Part print with two shaded views. Sizes in mm from the minimum x, y, z corner. Coordinates: 2 decimals unless noted, no trailing zeros. Loops run counter-clockwise (first coordinate to the right, second up) from the corner with the lowest first, then second, coordinate; pieces in that order, holes last. Notation, with made-up numbers: (41, 22.25) - (75, 22.25) arc R30 cw to (75, 61.25) - close; hole circle Ø10 at (9, 6.5). An arc over 180 degrees is marked (long way). Write each question's results on one line, items separated by ' | '. Start each with the question number.
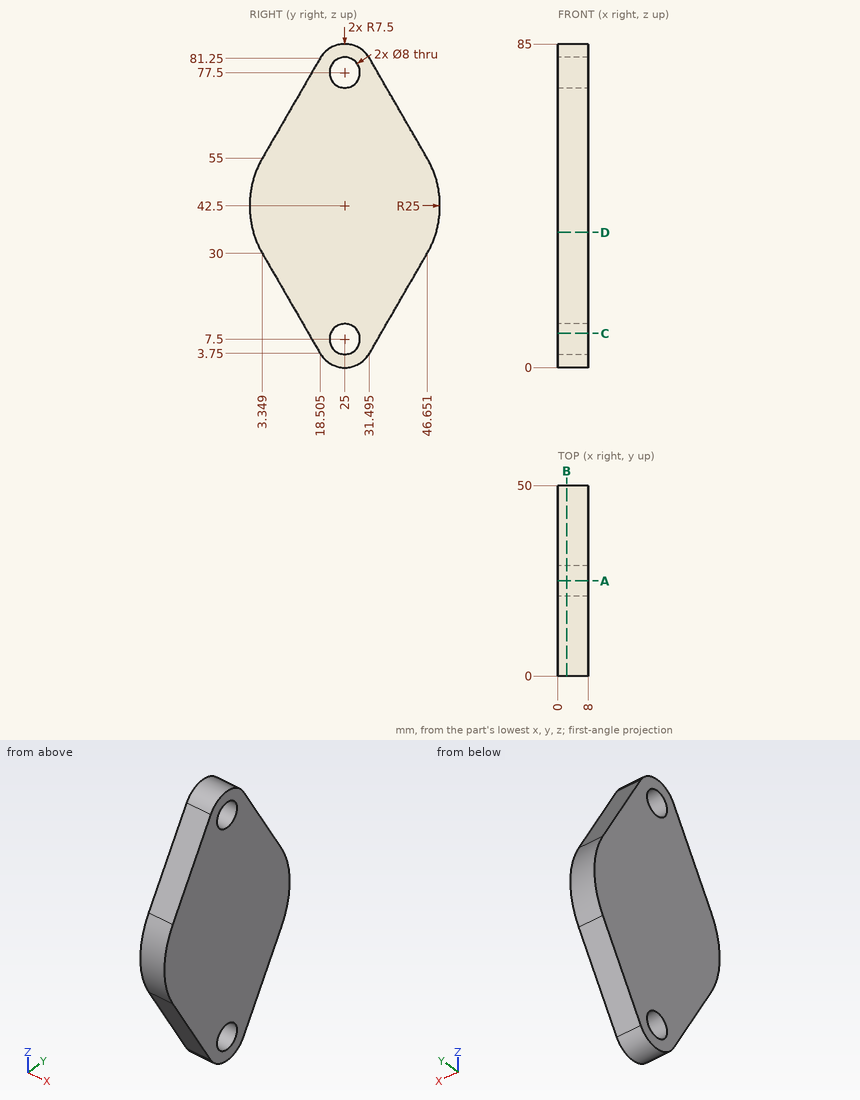
Q1. Cut at C-C (z = 9). List the corners of the cut face in (x, y), and give its area (3 significant figures).
Q2. Cut at B-B (x = 2.25). State how many separate pieces and enclosed holes the cut face has, and give its area (3 significant figures).
Q3. Cut at A-A (y = 25). List the corners of the cut face in (x, z).
Q4. Pin check, flat tips, straight feed: pin 1 (2 mm diameter, centred on x = 3, y = 43.5, fed in from +Z); pin 2 (2 mm diameter, centred on x = 1, z = 23, fed in from -Y); pin 3 (2 mm diameter, centred on x = 3.5, y = 13, fed in from +Z); pin 4 (10.5 mm diameter, centred on y = 25, z = 7.5, fed in from -X). Stop position of each tip, or through.
Q5. Drill centre lines: L1, parallel to Y at x = 5.75, z = 7.5; L2, parallel to Z at x = 2.5, y = 26.5; L3, parallel to Y at x = 4, z = 4.5 (1 decimal). Where is each one in solid material? Low to high. Write a range as from..to.
Q6. Cut at D-D (z = 35.5). List the corners of the cut face in (x, y).
Check result:
1) outline: (0, 15.47) - (8, 15.47) - (8, 21.29) - (0, 21.29) - close; (0, 28.71) - (8, 28.71) - (8, 34.53) - (0, 34.53) - close | area: 93.1 mm²
2) separate pieces: 1 | enclosed holes: 2 | area: 2,640 mm²
3) outline: (0, 0) - (8, 0) - (8, 3.5) - (0, 3.5) - close; (0, 11.5) - (8, 11.5) - (8, 73.5) - (0, 73.5) - close; (0, 81.5) - (8, 81.5) - (8, 85) - (0, 85) - close
4) pin 1: z = 62.19 | pin 2: y = 6.81 | pin 3: z = 73.45 | pin 4: x = 0
5) L1: 16.34..21, 29..33.66 | L2: 0.15..3.79, 11.21..73.79, 81.21..84.85 | L3: 18.1..22.4, 27.6..31.9
6) outline: (0, 1) - (8, 1) - (8, 49) - (0, 49) - close
